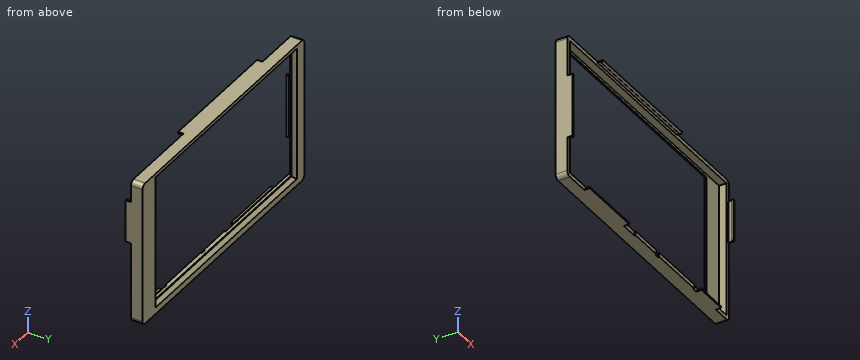
```python
from build123d import *

# Parameters (mm, degrees)
SKETCH_W      = 123
SKETCH_H      = 68
SKETCH_W_2    = 104
SKETCH_H_2    = 60
PAD_DEPTH     = 2
SKETCH001_W   = 123
SKETCH001_H   = 68
SKETCH001_W_2 = 119
SKETCH001_H_2 = 64
PAD001_DEPTH  = 3.5
PAD006_START  = -40
PAD006_DEPTH  = 60
PAD007_START  = -10
PAD007_DEPTH  = 20
PAD008_START  = -20
PAD008_DEPTH  = 30
PAD009_START  = -10
PAD009_DEPTH  = 15
PAD010_START  = -80
PAD010_DEPTH  = 30
SKETCH016_W   = 15.8
SKETCH016_H   = 2
SKETCH016_W_2 = 26.8
PAD014_DEPTH  = 0.5
FILLET_R      = 2
CHAMFER_SIZE  = 1.6


with BuildPart() as part:
    # Sketch → Pad (new body)
    with BuildSketch(Plane.XZ):
        with Locations((0.1, 0)):
            Rectangle(SKETCH_W, SKETCH_H)
        with Locations((-2, 0.7)):
            Rectangle(SKETCH_W_2, SKETCH_H_2, mode=Mode.SUBTRACT)
    extrude(amount=PAD_DEPTH)

    # Sketch001 (on Face10 of Pad) → Pad001 (join)
    with BuildSketch(Plane.XZ.offset(2)):
        with Locations((0.1, 0)):
            Rectangle(SKETCH001_W, SKETCH001_H)
        with Locations((0.1, 0)):
            Rectangle(SKETCH001_W_2, SKETCH001_H_2, mode=Mode.SUBTRACT)
    extrude(amount=PAD001_DEPTH)

    # Sketch008 (on Face7 of Pad001) → Pad006 (join)
    with BuildSketch(Plane(origin=(61.6, 0, 0), x_dir=(0, 0, 1), z_dir=(1, 0, 0)).offset(PAD006_START)):
        with BuildLine():
            Line((34, 5.5), (34, 8))
            Line((33.5, 8), (34, 8))
            ThreePointArc((33.5, 8), (33, 7.5), (33.5, 7))
            Line((33.5, 5.5), (33.5, 7))
            Line((33.5, 5.5), (34, 5.5))
        make_face()
    extrude(amount=-PAD006_DEPTH)

    # Sketch009 (on Face5 of Pad006) → Pad007 (join)
    with BuildSketch(Plane(origin=(0, 0, 34), x_dir=(-1, 0, 0), z_dir=(0, 0, 1)).offset(PAD007_START)):
        with BuildLine():
            Line((-61.1, 5.5), (-61.6, 5.5))
            Line((-61.6, 5.5), (-61.6, 8))
            Line((-61.6, 8), (-61.1, 8))
            ThreePointArc((-61.1, 7), (-60.6, 7.5), (-61.1, 8))
            Line((-61.1, 5.5), (-61.1, 7))
        make_face()
    extrude(amount=-PAD007_DEPTH)

    # Sketch010 (on Face5 of Pad007) → Pad008 (join)
    with BuildSketch(Plane(origin=(0, 0, 34), x_dir=(-1, 0, 0), z_dir=(0, 0, 1)).offset(PAD008_START)):
        with BuildLine():
            Line((60.9, 7), (60.9, 5.5))
            Line((60.9, 5.5), (61.4, 5.5))
            Line((61.4, 5.5), (61.4, 8))
            Line((61.4, 8), (60.9, 8))
            ThreePointArc((60.9, 8), (60.4, 7.5), (60.9, 7))
        make_face()
    extrude(amount=-PAD008_DEPTH)

    # Sketch011 (on Face7 of Pad008) → Pad009 (join)
    with BuildSketch(Plane(origin=(61.6, 0, 0), x_dir=(0, 0, 1), z_dir=(1, 0, 0)).offset(PAD009_START)):
        with BuildLine():
            Line((-33.5, 7), (-33.5, 5.5))
            Line((-33.5, 5.5), (-34, 5.5))
            Line((-34, 5.5), (-34, 8))
            Line((-34, 8), (-33.5, 8))
            ThreePointArc((-33.5, 7), (-33, 7.5), (-33.5, 8))
        make_face()
    extrude(amount=-PAD009_DEPTH)

    # Sketch011 (on Face7 of Pad008) → Pad010 (join)
    with BuildSketch(Plane(origin=(61.6, 0, 0), x_dir=(0, 0, 1), z_dir=(1, 0, 0)).offset(PAD010_START)):
        with BuildLine():
            Line((-33.5, 7), (-33.5, 5.5))
            Line((-33.5, 5.5), (-34, 5.5))
            Line((-34, 5.5), (-34, 8))
            Line((-34, 8), (-33.5, 8))
            ThreePointArc((-33.5, 7), (-33, 7.5), (-33.5, 8))
        make_face()
    extrude(amount=-PAD010_DEPTH)

    # Sketch016 (on Face13 of Pad010) → Pad014 (join)
    with BuildSketch(Plane.XZ.offset(5.5)):
        with Locations((-2.4, -33)):
            Rectangle(SKETCH016_W, SKETCH016_H)
        with Locations((21.1, -33)):
            Rectangle(SKETCH016_W_2, SKETCH016_H)
    extrude(amount=PAD014_DEPTH)

    # Fillet
    fillet_edges = [part.edges().sort_by_distance(p)[0] for p in [
        (61.6, -1, -34),
        (-61.4, -1, -34),
        (-61.4, -1, 34),
        (61.6, -1, 34),
    ]]
    fillet(fillet_edges, radius=FILLET_R)

    # Chamfer
    chamfer_edges = [part.edges().sort_by_distance(p)[0] for p in [
        (-54, 0, 0.7),
        (-2, 0, -29.3),
        (-2, 0, 30.7),
        (50, 0, 0.7),
    ]]
    chamfer(chamfer_edges, length=CHAMFER_SIZE)


solid = part.part
```
Source: CAD feature listing. Evaluate the final solid. Frame: model axes, mm. Give positions to 0.01 mm unless a question says otherwise; leave off trailing zeros. Loops run counter-clockwise (first coordinate to the right, second up) from the corner with the lowest first, then second, coordinate; pieces in that order, holes last. Notation, with made-up numbers: (-0.75, -34.5) -> (21.25, -34.5) arc R23 cw to (21.25, -19.5) -> close; hole circle Ø7 at (64.25, -9.5). An arc over 180 degrees is marked (long way). Put each result on its own line as item: value. Start each with the question number.
1) Cut plane C-C (z = -14). Return loops of the section in (x, y).
2) Cut plane D-D (x = -26). Return loops of the section in (y, z), then the cut area to 3 significant figures.
3) Contact query for flat-ended pins moving along their axis: P1, Ø0.8, axis at y = -6.5, z = 1.5, coming from the +X side; P2, Ø1, axis at x = -1.5, z = -33.5, coming from the -Y side; P3, Ø0.5, axis at y = -6.5, z = -33.5, coming from the +X side. Output: stop coordinate, or through.
4) Cut plane B-B (y = -3.5). Return loops of the section in (x, z), then the cut area to 3 significant figures.
5) Cut plane A-A (x = 43). Return loops of the section in (y, z), then the cut area to 3 significant figures.
6) Material intervals for probe 1 along X at (y, z) = (-2.75, 14); probe 2 along Z at (x, y) = (-20, -4.5); probe 3 along Z at (x, y) = (44, -6.25), sorted ascending.
Results are:
1. outline: (-61.4, -8) -> (-60.9, -8) arc R0.5 ccw to (-60.9, -7) -> (-60.9, -5.5) -> (-59.4, -5.5) -> (-59.4, -2) -> (-54, -2) -> (-54, -1.6) -> (-55.6, 0) -> (-61.4, 0) -> close; (50, -2) -> (59.6, -2) -> (59.6, -5.5) -> (61.6, -5.5) -> (61.6, 0) -> (51.6, 0) -> (50, -1.6) -> close
2. outline: (-8, -34) -> (0, -34) -> (0, -30.9) -> (-1.6, -29.3) -> (-2, -29.3) -> (-2, -32) -> (-5.5, -32) -> (-5.5, -33.5) -> (-7, -33.5) arc R0.5 ccw to (-8, -33.5) -> close; (-8, 33.5) arc R0.5 ccw to (-7, 33.5) -> (-5.5, 33.5) -> (-5.5, 32) -> (-2, 32) -> (-2, 30.7) -> (-1.6, 30.7) -> (0, 32.3) -> (0, 34) -> (-8, 34) -> close
2. area: 30.7 mm2
3. P1: stops at x = -60.9
3. P2: stops at y = -6
3. P3: stops at x = 51.6
4. outline: (-61.4, -32) arc R2 ccw to (-59.4, -34) -> (59.6, -34) arc R2 ccw to (61.6, -32) -> (61.6, 32) arc R2 ccw to (59.6, 34) -> (-59.4, 34) arc R2 ccw to (-61.4, 32) -> close; hole (-59.4, -32) -> (59.6, -32) -> (59.6, 32) -> (-59.4, 32) -> close
4. area: 745 mm2
5. outline: (-8, -34) -> (0, -34) -> (0, -30.9) -> (-1.6, -29.3) -> (-2, -29.3) -> (-2, -32) -> (-5.5, -32) -> (-5.5, -33.5) -> (-7, -33.5) arc R0.5 ccw to (-8, -33.5) -> close; (-5.5, 32) -> (-2, 32) -> (-2, 30.7) -> (-1.6, 30.7) -> (0, 32.3) -> (0, 34) -> (-5.5, 34) -> close
5. area: 29.1 mm2
6. probe 1: x = -61.4 to -59.4, 59.6 to 61.6
6. probe 2: z = -34 to -32, 32 to 34
6. probe 3: z = -34 to -33.5
